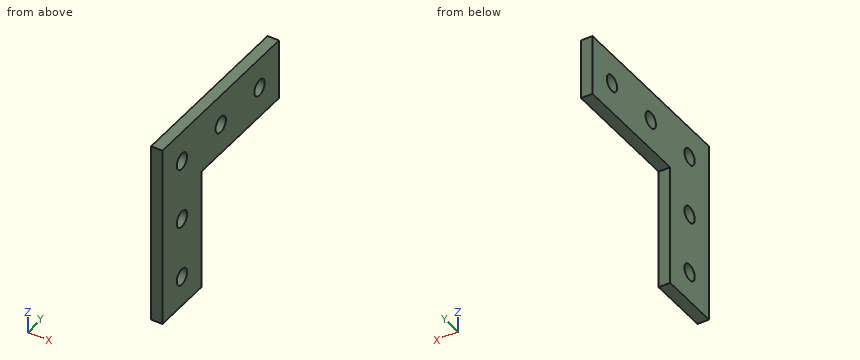
```python
from build123d import *

# Parameters (mm, degrees)
BOSS_EXTRUDE1_DEPTH         = 4.7752
F_1_4_CLEARANCE_HOLE1_D     = 6.7564
F_1_4_CLEARANCE_HOLE1_DEPTH = 14.478
F_1_4_CLEARANCE_HOLE1_TIP   = 2.029827343


with BuildPart() as part:
    # Sketch1 → Boss-Extrude1 (new body)
    with BuildSketch(Plane(origin=(0, 0, 0), x_dir=(0, 0, -1), z_dir=(1, 0, 0))):
        Polygon((0, 0), (0, 50.8), (-25.4, 50.8), (-25.4, -25.4), (50.8, -25.4), (50.8, 0), align=None)
    extrude(amount=BOSS_EXTRUDE1_DEPTH)

    # 1/4 Clearance Hole1
    with Locations(Plane(origin=(4.7752, 0, 0), x_dir=(0, 0, -1), z_dir=(1, 0, 0))):
        with Locations((-12.7, -12.7), (12.7, -12.7), (38.1, -12.7), (-12.7, 12.7), (-12.7, 38.1)):
            Hole(F_1_4_CLEARANCE_HOLE1_D / 2, depth=F_1_4_CLEARANCE_HOLE1_DEPTH)
            with Locations((0, 0, -(F_1_4_CLEARANCE_HOLE1_DEPTH + F_1_4_CLEARANCE_HOLE1_TIP / 2))):  # 118° drill point
                Cone(0, F_1_4_CLEARANCE_HOLE1_D / 2, F_1_4_CLEARANCE_HOLE1_TIP, mode=Mode.SUBTRACT)


solid = part.part
```
Read the model definition and answer for the solid it produces. Units are mm, in the model's axes. Coordinates: 2 decimals unless noted, no trailing zeros. Loops run counter-clockwise (first coordinate to the right, second up) from the corner with the lowest first, then second, coordinate; pieces in that order, holes last. Notation, with made-up numbers: (-23, 71) - (14, 71) arc R15 ccw to (14, 98) - close; hole circle Ø11 at (88, 53). An arc over 180 degrees is marked (long way). Answer in a Markdown table with one row per item.
1. Find section D-D, the plane z = -38.1. Write down the section's boundary in (x, y).
Conclusion:
| item | result |
|---|---|
| outline | (0, -25.4) - (4.78, -25.4) - (4.78, -16.08) - (0, -16.08) - close; (0, -9.32) - (4.78, -9.32) - (4.78, 0) - (0, 0) - close |
2. Find section A-A, the plane z = 12.7. Write down the section's boundary in (x, y).
Conclusion:
| item | result |
|---|---|
| outline | (0, -25.4) - (4.78, -25.4) - (4.78, -16.08) - (0, -16.08) - close; (0, -9.32) - (4.78, -9.32) - (4.78, 9.32) - (0, 9.32) - close; (0, 16.08) - (4.78, 16.08) - (4.78, 34.72) - (0, 34.72) - close; (0, 41.48) - (4.78, 41.48) - (4.78, 50.8) - (0, 50.8) - close |
3. Find section C-C, the plane y = -12.7. Write down the section's boundary in (x, z), then the cut area to 3 significant figures.
Conclusion:
| item | result |
|---|---|
| outline | (0, -50.8) - (4.78, -50.8) - (4.78, -41.48) - (0, -41.48) - close; (0, -34.72) - (4.78, -34.72) - (4.78, -16.08) - (0, -16.08) - close; (0, -9.32) - (4.78, -9.32) - (4.78, 9.32) - (0, 9.32) - close; (0, 16.08) - (4.78, 16.08) - (4.78, 25.4) - (0, 25.4) - close |
| area | 267 mm² |
4. Given pin 1 (1.5 mm diameter, centred on x = 3, z = -42.5, fed in from +Y); pin 2 (9 mm diameter, centred on y = 12.7, z = 12.7, fed in from -X), each flat-ended and moving along its own axis, determine where each tip first touches the part or whether it passes through.
Conclusion:
| item | result |
|---|---|
| pin 1 | stops at y = 0 |
| pin 2 | stops at x = 0 |
5. Find section B-B, the plane x = 1.55. Write down the section's boundary in (y, z).
Conclusion:
| item | result |
|---|---|
| outline | (-25.4, -50.8) - (0, -50.8) - (0, 0) - (50.8, 0) - (50.8, 25.4) - (-25.4, 25.4) - close; hole circle Ø6.76 at (-12.7, -38.1); hole circle Ø6.76 at (-12.7, -12.7); hole circle Ø6.76 at (-12.7, 12.7); hole circle Ø6.76 at (12.7, 12.7); hole circle Ø6.76 at (38.1, 12.7) |
6. Straight lines are drawn through the part: line 1 (Y direction, x = 3.5, z = 12.7); line 2 (Y direction, x = 1.35, z = -12.7); line 3 (Y direction, x = 0.85, z = -20). For each, find the intervals that lie inside material, in ascending order.
Conclusion:
| item | result |
|---|---|
| line 1 | y = -25.4 to -16.08, -9.32 to 9.32, 16.08 to 34.72, 41.48 to 50.8 |
| line 2 | y = -25.4 to -16.08, -9.32 to 0 |
| line 3 | y = -25.4 to 0 |
